```python
from build123d import *

# Parameters (mm, degrees)
SKETCH1_W           = 90
SKETCH1_H           = 110
BOSS_EXTRUDE1_DEPTH = 28
FILLET2_R           = 30
SKETCH3_R           = 1.5
CUT_EXTRUDE1_DEPTH  = 145.858551698
SKETCH4_R           = 3
CUT_EXTRUDE4_DEPTH  = 26
CUT_EXTRUDE5_START  = -13.7
SKETCH5_W           = 73
SKETCH5_H           = 87
CUT_EXTRUDE5_DEPTH  = 13.7
CUT_EXTRUDE5_TAPER  = 15
SKETCH8_W           = 73
SKETCH8_H           = 87
CUT_EXTRUDE8_DEPTH  = 11.8
CUT_EXTRUDE8_DRAFT  = -70
CUT_EXTRUDE9_START  = 30
SKETCH9_R           = 11.28
CUT_EXTRUDE9_DEPTH  = 61.8
FILLET19_R          = 20
SKETCH13_W          = 90
SKETCH13_H          = 55
CUT_EXTRUDE10_DEPTH = 145.858551855
CUT_EXTRUDE12_REACH = 146.859
SKETCH15_W          = 5
SKETCH15_H          = 55
CUT_EXTRUDE13_DEPTH = 145.858551855


with BuildPart() as part:
    # Sketch1 → Boss-Extrude1 (new body)
    with BuildSketch(Plane.XY):
        with Locations((45, 55)):
            Rectangle(SKETCH1_W, SKETCH1_H)
    extrude(amount=BOSS_EXTRUDE1_DEPTH)

    # Fillet2
    # the kernel refuses this fillet: 30 mm, written as the material it takes off along each edge
    with BuildSketch(Plane(origin=(-74.833147735, 0, 28), x_dir=(0, 0, -1), z_dir=(1, 0, 0)), Plane(origin=(164.833147735, 110, 28), x_dir=(0, 0, -1), z_dir=(-1, 0, 0))) as fillet2_piece_1:
        with BuildLine():
            CenterArc((30, 29.933259094), FILLET2_R, 180, 86.177446271)
            Line((0, 29.933259094), (-0.6, 29.933259094))
            Line((-0.6, 29.933259094), (-0.6, 0))
            Line((-0.6, 0), (0, -0.6))
            ThreePointArc((0, -0.6), (14, -0.6), (27.96, -0.598665182))
            Line((27.96, -0.598665182), (28, 0))
        make_face()
    extrude(amount=239.666295471, mode=Mode.SUBTRACT)

    # Sketch3 → Cut-Extrude1 (cut, through all)
    with BuildSketch(Plane(origin=(0, 0, 0), x_dir=(-1, 0, 0), z_dir=(0, 0, -1))):
        with Locations((-45, 105)):
            Circle(SKETCH3_R)
        with Locations((-45, 5)):
            Circle(SKETCH3_R)
        with Locations((-5, 70)):
            Circle(SKETCH3_R)
        with Locations((-5, 40)):
            Circle(SKETCH3_R)
    extrude(amount=-CUT_EXTRUDE1_DEPTH, mode=Mode.SUBTRACT)

    # Sketch4 → Cut-Extrude4 (cut)
    with BuildSketch(Plane.XY.offset(28)):
        with Locations((45, 105)):
            Circle(SKETCH4_R)
        with Locations((45, 5)):
            Circle(SKETCH4_R)
        with Locations((5, 70)):
            Circle(SKETCH4_R)
        with Locations((5, 40)):
            Circle(SKETCH4_R)
    extrude(amount=-CUT_EXTRUDE4_DEPTH, mode=Mode.SUBTRACT)

    # Sketch5 → Cut-Extrude5 (cut)
    with BuildSketch(Plane(origin=(0, 0, 0), x_dir=(-1, 0, 0), z_dir=(0, 0, -1)).offset(CUT_EXTRUDE5_START)):
        with Locations((-45, 55)):
            Rectangle(SKETCH5_W, SKETCH5_H)
    extrude(amount=CUT_EXTRUDE5_DEPTH, taper=CUT_EXTRUDE5_TAPER, mode=Mode.SUBTRACT)


with BuildPart() as cut_extrude8_tool:
    # Sketch8 → Cut-Extrude8 (with draft: the straight prism first)
    with BuildSketch(Plane(origin=(0, 0, 13.7), x_dir=(-1, 0, 0), z_dir=(0, 0, -1))):
        with Locations((-45, 55)):
            Rectangle(SKETCH8_W, SKETCH8_H)
    extrude(amount=-CUT_EXTRUDE8_DEPTH)
    # Cut-Extrude8: the draft: its side faces are tilted about the plane it starts from
    cut_extrude8_sides = [cut_extrude8_tool.faces().sort_by_distance(p)[0] for p in [
        (81.5, 55, 19.6),
        (45, 11.5, 19.6),
        (8.5, 55, 19.6),
        (45, 98.5, 19.6),
    ]]
    draft(cut_extrude8_sides, Plane(origin=(0, 0, 13.7), x_dir=(-1, 0, 0), z_dir=(0, 0, -1)), CUT_EXTRUDE8_DRAFT)


with BuildPart() as part_1:
    add(part.part)

    # Cut-Extrude8: cut by cut_extrude8_tool
    add(cut_extrude8_tool.part, mode=Mode.SUBTRACT)

    # Sketch9 → Cut-Extrude9 (cut)
    with BuildSketch(Plane(origin=(0, 0, 25.5), x_dir=(-1, 0, 0), z_dir=(0, 0, -1)).offset(CUT_EXTRUDE9_START)):
        with Locations((-45.00023355, 55.00023355)):
            Circle(SKETCH9_R)
    extrude(amount=-CUT_EXTRUDE9_DEPTH, mode=Mode.SUBTRACT)

    # Fillet19
    fillet19_edges = [part_1.edges().sort_by_distance(p)[0] for p in [
        (79.664548032, 96.664548032, 6.85),
        (79.664548032, 13.335451968, 6.85),
        (10.335451968, 13.335451968, 6.85),
        (10.335451968, 96.664548032, 6.85),
    ]]
    fillet(fillet19_edges, radius=FILLET19_R)

    # Sketch13 → Cut-Extrude10 (cut, through all)
    with BuildSketch(Plane(origin=(0, 0, 0), x_dir=(-1, 0, 0), z_dir=(0, 0, -1))):
        with Locations((-45, 27.5)):
            Rectangle(SKETCH13_W, SKETCH13_H)
    extrude(amount=-CUT_EXTRUDE10_DEPTH, mode=Mode.SUBTRACT)

    # Cut-Extrude12: up to this plane
    cut_extrude12_end = Plane(origin=(8.5, 11.5, 13.7), z_dir=(-0.9659258262890681, 0, -0.25881904510252135))
    # Sketch14 → Cut-Extrude12 (cut, up to the surface)
    with BuildSketch(Plane.ZY, mode=Mode.PRIVATE) as cut_extrude12_sk1:
        with BuildLine():
            Line((6.5, 58.5), (0, 58.5))
            Line((0, 58.5), (0, 51.5))
            Line((0, 51.5), (6.5, 51.5))
            ThreePointArc((6.5, 51.5), (10, 55), (6.5, 58.5))
        make_face()
    cut_extrude12_tool1 = split(extrude(cut_extrude12_sk1.sketch, amount=-CUT_EXTRUDE12_REACH, mode=Mode.PRIVATE), bisect_by=cut_extrude12_end, keep=Keep.BOTH, mode=Mode.PRIVATE)
    add(cut_extrude12_tool1.solids().sort_by_distance((0, 55, 4.657437))[0], mode=Mode.SUBTRACT)

    # Sketch15 → Cut-Extrude13 (cut, through all)
    with BuildSketch(Plane(origin=(0, 0, 0), x_dir=(-1, 0, 0), z_dir=(0, 0, -1))):
        with Locations((-87.5, 82.5)):
            Rectangle(SKETCH15_W, SKETCH15_H)
    extrude(amount=-CUT_EXTRUDE13_DEPTH, mode=Mode.SUBTRACT)


solid = part_1.part
```
Can you work these out from the model? Positions are in its coordinate system, mm. A direction names the side the tool comes from. Coordinates: 2 decimals unless noted, no trailing zeros. Order: outer loops, then holes, each group sorted by start corner. A loop starts at its lowest first (then second) coordinate and runs counter-clockwise, first axis right, second up.
1. For faces 1 (the face through (44.35, 102.07, 8.52)), 2 (the face through (6, 58.5, 3)), 3 (the face through (20.881, 69.67, 18.206)), which set-ups out of +Z, -Z, +X, -X, +Y, -Y let a thin tool reach every point of the face, with its end or its side?
2. If we section it at A-A (y = 105): Please give me the cut outline in (x, z).
3. If we section it at B-B (z = 8.5): Give the number of separate pieces and of enclosed holes in the cut face, then the cut area to 3 significant figures.
4. Thinking about a two-plate mould opening in Y: for faces 4 (the face through (4.35, 67.07, 15.18)), 5 (the face through (43.1, 100.33, 20.12)), 6 (the face through (69.119, 69.67, 18.206)), which applies, +Y half, -Y half, draft (parallel to the pull), parting line (faces both ways), or undercut?
5. I'm going to push flat-ended pins straight in: pin 1 (6 mm diameter, centred on x = 49, z = 13, fed in from +Y); pin 2 (1 mm diameter, centred on x = 43.5, y = 83, fed in from -Z); pin 3 (5 mm diameter, centred on x = 50.5, y = 66, fed in from -Z); pin 4 (2.5 mm diameter, centred on x = 45, y = 105, fed in from +Z). Where does each tip first touch, or does it pass through?
6. I need wall thicknesses on line 1 (X direction, y = 105, z = 12.75); line 2 (X direction, y = 72.5, z = 8); line 3 (X direction, y = 105, z = 1.2). Which ranges of each line are inside material? Lowest first, please.
Entries:
1. face 1: +Z
1. face 2: -Z, -X, -Y
1. face 3: -Y
2. outline: (0, 0) - (43.5, 0) - (43.5, 2) - (42, 2) - (42, 14.68) - (0, 14.68) - close; (46.5, 0) - (85, 0) - (85, 14.68) - (48, 14.68) - (48, 2) - (46.5, 2) - close
3. separate pieces: 1
3. enclosed holes: 2
3. area: 1,630 mm2
4. face 4: undercut
4. face 5: +Y half
4. face 6: draft
5. pin 1: stops at y = 107.56
5. pin 2: stops at z = 19.16
5. pin 3: stops at z = 24.07
5. pin 4: passes through
6. line 1: x = 0 to 42, 48 to 85
6. line 2: x = 0 to 3.34, 6.66 to 10.03, 79.97 to 85
6. line 3: x = 0 to 43.5, 46.5 to 85
